Design review of the part shown in the three views and the two pictorial views. Dimensions are in mm from the part's minimum x, y and z. A direction names the side the tool comes from. Coordinates: 2 decimals unless noted, no trailing zeros. Order: outer loops, then holes, each group sorted by start corner. A loop starts at its lowest first (then second) coordinate and runs counter-clockwise, first axis right, second up. Notation, with made-up numbers: (-34.75, 49) - (17.25, 49) arc R4 ccw to (17.25, 53) - close; hole circle Ø11 at (-7.5, 41). An arc over 180 degrees is marked (long way). One line per item, written item: value. Start each with the question number.
(1) Consider section B-B on x = 24.25. Write out the cut boundary in (y, z), then the cut area to 3 significant figures.
(2) To check wall thickness, follow line 1 along Z through (x, y) = (24, 1.1); line 2 along X through (y, z) = (0.55, 5.75); line 3 along X through (y, z) = (1.85, 8.75). State the ranges of each line that lie inside material, in increasing order.
(3) Consider section A-A on y = 2.8. Write out the cut boundary in (x, z), then the cut area to 3 significant figures.
(4) Clearance check with a flat-ended pin moving along its axis: pin 1 (2 mm diameter, centred on x = 4.5, y = 1, fed in from +Z). State where the tip first meets the part, or that it passes through.
(5) For the marked faces 1, 2 and 3, list the 3-axis set-ups (+Z, -Z, +X, -X, +Y, -Y) from which the entire face can be reached by the end or side of a thin tool; tool diameter is ignored.
(6) Consider section C-C on z = 11. Write out the cut boundary in (x, y).
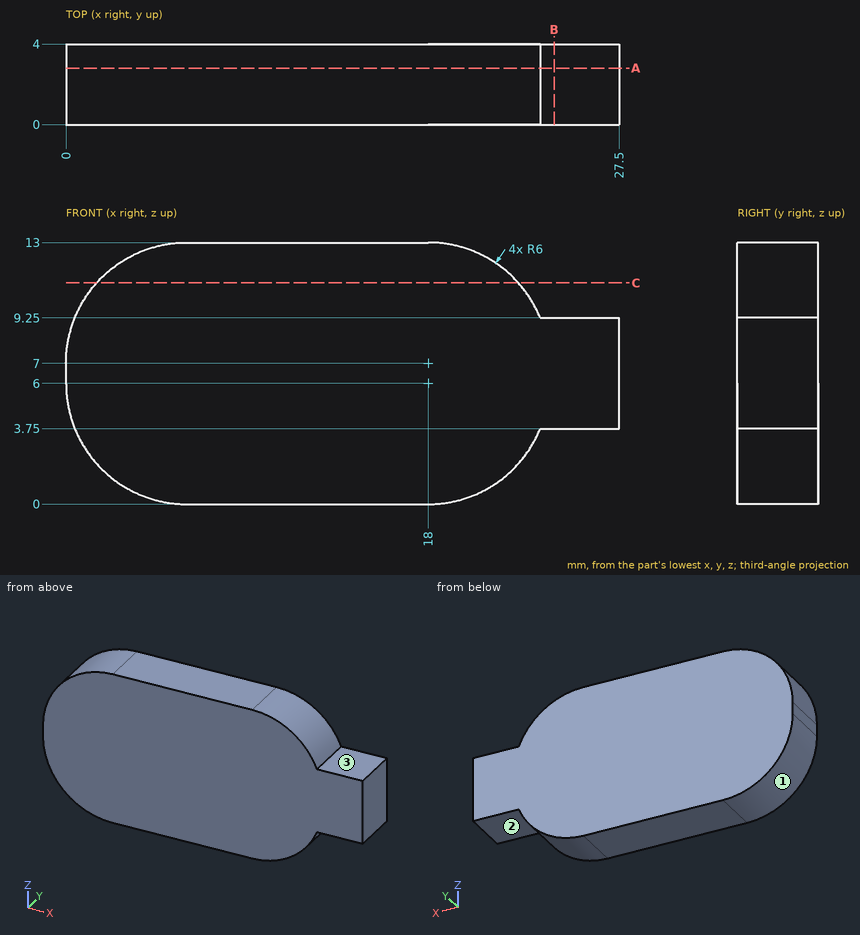
Geometry check:
1. outline: (0, 3.75) - (4, 3.75) - (4, 9.25) - (0, 9.25) - close
1. area: 22.0 mm^2
2. line 1: z = 3.75 to 9.25
2. line 2: x = 0.01 to 27.5
2. line 3: x = 0.26 to 27.5
3. outline: (0, 6) arc R6 ccw to (6, 0) - (18, 0) arc R6 ccw to (23.56, 3.75) - (27.5, 3.75) - (27.5, 9.25) - (23.56, 9.25) arc R6 ccw to (18, 13) - (6, 13) arc R6 ccw to (0, 7) - close
3. area: 301 mm^2
4. pin 1: stops at z = 12.98
5. face 1: -Z, -X, +Y, -Y
5. face 2: -Z, +X, +Y, -Y
5. face 3: +Z, +X, +Y, -Y
6. outline: (1.53, 0) - (22.47, 0) - (22.47, 4) - (1.53, 4) - close
